Read the model definition and answer for the solid it produces. Units are mm, in the model's axes. A direction names the side the tool comes from. Coordinates: 2 decimals unless noted, no trailing zeros. Loops run counter-clockwise (first coordinate to the right, second up) from the corner with the lowest first, then second, coordinate; pieces in that order, holes last.
from build123d import *

# Parameters (mm, degrees)
CROQUIS1_W              = 15
CROQUIS1_H              = 100
CROQUIS1_R              = 1.25
SALIENTE_EXTRUIR1_DEPTH = 2
CROQUIS2_W              = 10
CROQUIS2_H              = 15
SALIENTE_EXTRUIR2_DEPTH = 9


with BuildPart() as part:
    # Croquis1 → Saliente-Extruir1 (new body)
    with BuildSketch(Plane.XY):
        Rectangle(CROQUIS1_W, CROQUIS1_H)
        with Locations((0, 42.5)):
            Circle(CROQUIS1_R, mode=Mode.SUBTRACT)
        with Locations((0, 17.5)):
            Circle(CROQUIS1_R, mode=Mode.SUBTRACT)
        with Locations((0, -42.5)):
            Circle(CROQUIS1_R, mode=Mode.SUBTRACT)
        with Locations((0, -17.5)):
            Circle(CROQUIS1_R, mode=Mode.SUBTRACT)
    extrude(amount=-SALIENTE_EXTRUIR1_DEPTH)

    # Croquis2 → Saliente-Extruir2 (add)
    with BuildSketch(Plane.XY):
        with Locations((0, 30)):
            Rectangle(CROQUIS2_W, CROQUIS2_H)
        with Locations((0, -30)):
            Rectangle(CROQUIS2_W, CROQUIS2_H)
    extrude(amount=SALIENTE_EXTRUIR2_DEPTH)


solid = part.part
Item 1: A cutting plane is placed at B-B on x = 0. Determine the outline of the cut face in (y, z), then the cut area to 3 significant figures.
Numbers:
outline: (-50, -2) - (-43.75, -2) - (-43.75, 0) - (-50, 0) - close; (-41.25, -2) - (-18.75, -2) - (-18.75, 0) - (-22.5, 0) - (-22.5, 9) - (-37.5, 9) - (-37.5, 0) - (-41.25, 0) - close; (-16.25, -2) - (16.25, -2) - (16.25, 0) - (-16.25, 0) - close; (18.75, -2) - (41.25, -2) - (41.25, 0) - (37.5, 0) - (37.5, 9) - (22.5, 9) - (22.5, 0) - (18.75, 0) - close; (43.75, -2) - (50, -2) - (50, 0) - (43.75, 0) - close
area: 450 mm2
Item 2: Which of the six approach directions +Z, -Z, +X, -X, +Y, -Y give full straight-line access (tool end or side, diameter ignored) to faces 1 (the face through (5, 30, 4)), 2 (the face through (0, -37.5, 4)), 3 (the face through (0, 22.5, 4)), 4 (the face through (-5, -30, 4))?
Numbers:
face 1: +Z, +X, +Y, -Y
face 2: +Z, +X, -X, -Y
face 3: +Z, +X, -X
face 4: +Z, -X, +Y, -Y
Item 3: A cutting plane is placed at D-D on x = 3.75. Determine the outline of the cut face in (y, z), then the cut area to 3 significant figures.
Numbers:
outline: (-50, -2) - (50, -2) - (50, 0) - (37.5, 0) - (37.5, 9) - (22.5, 9) - (22.5, 0) - (-22.5, 0) - (-22.5, 9) - (-37.5, 9) - (-37.5, 0) - (-50, 0) - close
area: 470 mm2
Item 4: A cutting plane is placed at C-C on y = -42.5. Determine the outline of the cut face in (x, z).
Numbers:
outline: (-7.5, -2) - (-1.25, -2) - (-1.25, 0) - (-7.5, 0) - close; (1.25, -2) - (7.5, -2) - (7.5, 0) - (1.25, 0) - close
Item 5: Find the intervals of material crossed by line 1 along Y through (x, z) = (0, -1.35); line 2 along Y through (x, z) = (-4.5, 2); line 3 along Z through (x, y) = (5.75, -32), in increasing order.
Numbers:
line 1: y = -50 to -43.75, -41.25 to -18.75, -16.25 to 16.25, 18.75 to 41.25, 43.75 to 50
line 2: y = -37.5 to -22.5, 22.5 to 37.5
line 3: z = -2 to 0
Item 6: A cutting plane is placed at A-A on z = 2.25. Determine the outline of the cut face in (x, y).
Numbers:
outline: (-5, -37.5) - (5, -37.5) - (5, -22.5) - (-5, -22.5) - close; (-5, 22.5) - (5, 22.5) - (5, 37.5) - (-5, 37.5) - close
Item 7: Given pin 1 (3 mm diameter, centred on x = 0, y = -42.5, fed in from +Z); pin 2 (5 mm diameter, centred on x = -2.5, z = 5.5, fed in from -Y); pin 3 (4.5 mm diameter, centred on x = -1.5, z = 5, fed in from +Y); pin 4 (1.5 mm diameter, centred on x = 0, y = -17.5, fed in from -Z), each flat-ended and moving along its own axis, determine where each tip first touches the part or whether it passes through.
Numbers:
pin 1: stops at z = 0
pin 2: stops at y = -37.5
pin 3: stops at y = 37.5
pin 4: passes through
Item 8: Determine the mould class of faces 5 (the face through (5, -30, 4)), 6 (the face through (-5, 30, 4)), 7 (the face through (-0.27, 16.28, -0.99)), 8 (the face through (0, 1, 0)) for opening direction X: released by +X, released by -X, zero draft, split by the parting line, or undercut.
Numbers:
face 5: released by +X
face 6: released by -X
face 7: undercut
face 8: zero draft
